from build123d import *

# Parameters (mm, degrees)
SKETCH_2_W          = 80.1
SKETCH_2_H          = 60.1
EXTRUDE_1_DEPTH     = 28
CUT_EXTRUDE_1_DEPTH = 106
SKETCH_6_R          = 1.8
CUT_EXTRUDE_2_DEPTH = 106
CUT_EXTRUDE_3_DEPTH = 92
FILLET_2_R          = 2
FILLET_3_R          = 10
FILLET_4_R          = 2


with BuildPart() as part:
    # 草图2 → 凸台-拉伸1 (new body)
    with BuildSketch(Plane.XY):
        with Locations((40.05, -30.05)):
            Rectangle(SKETCH_2_W, SKETCH_2_H)
    extrude(amount=EXTRUDE_1_DEPTH)

    # 草图3 → 切除-拉伸1 (cut)
    with BuildSketch(Plane.ZY):
        with BuildLine():
            ThreePointArc((14, -22), (6.928932188, -24.928932188), (4, -32))
            Line((4, -32), (14, -32))
            Line((14, -32), (14, -22))
        make_face()
        with BuildLine():
            Line((14, -32), (4, -32))
            ThreePointArc((4, -32), (6.928932188, -39.071067812), (14, -42))
            Line((14, -42), (14, -32))
        make_face()
        with BuildLine():
            Line((14, -22), (14, -32))
            Line((14, -32), (24, -32))
            ThreePointArc((24, -32), (21.071067812, -24.928932188), (14, -22))
        make_face()
        with BuildLine():
            Line((24, -32), (14, -32))
            Line((14, -32), (14, -42))
            ThreePointArc((14, -42), (21.071067812, -39.071067812), (24, -32))
        make_face()
    extrude(amount=-CUT_EXTRUDE_1_DEPTH, mode=Mode.SUBTRACT)

    # 草图6 → 切除-拉伸2 (cut)
    with BuildSketch(Plane.XY.offset(28)):
        with Locations((21.05, -3)):
            Circle(SKETCH_6_R)
        with Locations((59.05, -3)):
            Circle(SKETCH_6_R)
        with Locations((10.05, -54.5)):
            Circle(SKETCH_6_R)
        with Locations((70.05, -54.5)):
            Circle(SKETCH_6_R)
    extrude(amount=-CUT_EXTRUDE_2_DEPTH, mode=Mode.SUBTRACT)

    # 草图9 → 切除-拉伸3 (cut)
    with BuildSketch(Plane(origin=(0, 0, 0), x_dir=(1, 0, 0), z_dir=(0, 1, 0))):
        Polygon((0, 0), (0, -11.5), (25.05, -11.5), (25.05, -16.5), (55.05, -16.5), (55.05, -11.5), (80.1, -11.5), (80.1, 0), align=None)
    extrude(amount=-CUT_EXTRUDE_3_DEPTH, mode=Mode.SUBTRACT)

    # 圆角2
    fillet_2_edges = [part.edges().sort_by_distance(p)[0] for p in [
        (55.05, -50.891229183, 11.5),
        (55.05, -11.158770817, 11.5),
        (55.05, -50.891229183, 16.5),
        (55.05, -11.158770817, 16.5),
        (25.05, -50.891229183, 16.5),
        (25.05, -11.158770817, 16.5),
        (25.05, -50.891229183, 11.5),
        (25.05, -11.158770817, 11.5),
    ]]
    fillet(fillet_2_edges, radius=FILLET_2_R)

    # 圆角3
    fillet_3_edges = [part.edges().sort_by_distance(p)[0] for p in [
        (80.1, -60.1, 19.75),
        (0, -60.1, 19.75),
        (0, 0, 19.75),
        (80.1, 0, 19.75),
    ]]
    fillet(fillet_3_edges, radius=FILLET_3_R)

    # 圆角4
    # the kernel refuses this fillet: 2 mm, written as the material it takes off along each edge
    with BuildSketch(Plane(origin=(0, -50.1, 28), x_dir=(0, 0, -1), z_dir=(0, 1, 0))) as fillet_4_piece_1:
        with BuildLine():
            CenterArc((FILLET_4_R, -FILLET_4_R), FILLET_4_R, 90, 90)
            Line((0, -FILLET_4_R), (0, 0))
            Line((0, 0), (FILLET_4_R, 0))
        make_face()
    extrude(amount=40.1, mode=Mode.SUBTRACT)
    with BuildSketch(Plane(origin=(10, 0, 28), x_dir=(0, -1, 0), z_dir=(1, 0, 0))) as fillet_4_piece_2:
        with BuildLine():
            CenterArc((FILLET_4_R, FILLET_4_R), FILLET_4_R, 180, 90)
            Line((0, FILLET_4_R), (0, 0))
            Line((0, 0), (FILLET_4_R, 0))
        make_face()
    extrude(amount=60.1, mode=Mode.SUBTRACT)
    with BuildSketch(Plane(origin=(80.1, -10, 28), x_dir=(-1, 0, 0), z_dir=(0, -1, 0))) as fillet_4_piece_3:
        with BuildLine():
            CenterArc((FILLET_4_R, FILLET_4_R), FILLET_4_R, 180, 90)
            Line((0, FILLET_4_R), (0, 0))
            Line((0, 0), (FILLET_4_R, 0))
        make_face()
    extrude(amount=40.1, mode=Mode.SUBTRACT)
    with BuildSketch(Plane(origin=(70.1, -60.1, 28), x_dir=(0, 0, -1), z_dir=(-1, 0, 0))) as fillet_4_piece_4:
        with BuildLine():
            CenterArc((FILLET_4_R, -FILLET_4_R), FILLET_4_R, 90, 90)
            Line((0, -FILLET_4_R), (0, 0))
            Line((0, 0), (FILLET_4_R, 0))
        make_face()
    extrude(amount=60.1, mode=Mode.SUBTRACT)
    with BuildSketch(Plane(origin=(70.1, -10, 28), x_dir=(1, 0, 0), z_dir=(0, -1, 0))) as fillet_4_piece_5:
        with BuildLine():
            CenterArc((10 - FILLET_4_R, -FILLET_4_R), FILLET_4_R, 0, 90)
            Line((10, -FILLET_4_R), (10, 0))
            Line((10, 0), (10 - FILLET_4_R, 0))
        make_face()
    revolve(axis=Axis((70.1, -10, 28), (0, 0, 1)), revolution_arc=90, mode=Mode.SUBTRACT)
    with BuildSketch(Plane(origin=(70.1, -50.1, 28), x_dir=(1, 0, 0), z_dir=(0, 1, 0))) as fillet_4_piece_6:
        with BuildLine():
            CenterArc((10 - FILLET_4_R, FILLET_4_R), FILLET_4_R, 270, 90)
            Line((10, FILLET_4_R), (10, 0))
            Line((10, 0), (10 - FILLET_4_R, 0))
        make_face()
    revolve(axis=Axis((70.1, -50.1, 28), (0, 0, -1)), revolution_arc=90, mode=Mode.SUBTRACT)
    with BuildSketch(Plane(origin=(10, -50.1, 28), x_dir=(-1, 0, 0), z_dir=(0, 1, 0))) as fillet_4_piece_7:
        with BuildLine():
            CenterArc((10 - FILLET_4_R, -FILLET_4_R), FILLET_4_R, 0, 90)
            Line((10 - FILLET_4_R, 0), (10, 0))
            Line((10, 0), (10, -FILLET_4_R))
        make_face()
    revolve(axis=Axis((10, -50.1, 28), (0, 0, 1)), revolution_arc=90, mode=Mode.SUBTRACT)
    with BuildSketch(Plane(origin=(10, -10, 28), x_dir=(-1, 0, 0), z_dir=(0, -1, 0))) as fillet_4_piece_8:
        with BuildLine():
            CenterArc((10 - FILLET_4_R, FILLET_4_R), FILLET_4_R, 270, 90)
            Line((10, FILLET_4_R), (10, 0))
            Line((10, 0), (10 - FILLET_4_R, 0))
        make_face()
    revolve(axis=Axis((10, -10, 28), (0, 0, -1)), revolution_arc=90, mode=Mode.SUBTRACT)


solid = part.part
Geometry: final body of the model. Coordinates: model frame, mm. A direction names the side the tool comes from. Give positions to 0.01 mm unless a question says otherwise; leave off trailing zeros. Loops run counter-clockwise (first coordinate to the right, second up) from the corner with the lowest first, then second, coordinate; pieces in that order, holes last. Notation, with made-up numbers: (12, -24.5) -> (23, -24.5) arc R23 cw to (23, -13.5) -> close; hole circle Ø11 at (-14, 30.25). An arc over 180 degrees is marked (long way). Put each result on its own line as item: value.
1. Set-up query: faces 5 (the flat face through (0, -26, 23)), 6 (the cylindrical face through (25.62, -51.02, 15.9)). Return all of +Z, -Z, +X, -X, +Y, -Y with unobstructed straight access to the full face (end or side cutting, diameter ignored); none if empty.
Taken from the geometry:
face 5: +Z, -Z, -X, +Y, -Y
face 6: -Z, +Y, -Y
2. Cut plane B-B (x = 40.5). Return the cut outline in (y, z), plus the area to 3 significant figures.
Taken from the geometry:
outline: (-60.1, 16.5) -> (-41.68, 16.5) arc R10 cw to (-22.32, 16.5) -> (0, 16.5) -> (0, 26) arc R2 ccw to (-2, 28) -> (-58.1, 28) arc R2 ccw to (-60.1, 26) -> close
area: 582 mm2
3. Cut plane C-C (y = -16). Return the cut outline in (x, z).
Taken from the geometry:
outline: (0, 11.5) -> (23.05, 11.5) arc R2 ccw to (25.05, 13.5) -> (25.05, 14.5) arc R2 cw to (27.05, 16.5) -> (53.05, 16.5) arc R2 cw to (55.05, 14.5) -> (55.05, 13.5) arc R2 ccw to (57.05, 11.5) -> (80.1, 11.5) -> (80.1, 26) arc R2 ccw to (78.1, 28) -> (2, 28) arc R2 ccw to (0, 26) -> close
4. Pin query (flat end, axial travel): P1, Ø5.5, axis at x = 35, y = -54.5, coming from the -Z side; P2, Ø1, axis at x = 8.5, z = 16, coming from the +Y side; P3, Ø1.1, axis at y = -53.5, z = 14, coming from the +X side. Return the tip coordinate at first contact, or that it passes through.
Taken from the geometry:
P1: stops at z = 16.5
P2: stops at y = -0.05
P3: stops at x = 79.69
5. Cut plane D-D (z = 15.5). Return the cut outline in (x, y).
Taken from the geometry:
outline: (0, -50.1) arc R10 ccw to (10, -60.1) -> (25.32, -60.1) -> (25.32, -41.89) -> (0, -41.89) -> close; (0, -22.11) -> (25.32, -22.11) -> (25.32, 0) -> (10, 0) arc R10 ccw to (0, -10) -> close; (54.78, -60.1) -> (70.1, -60.1) arc R10 ccw to (80.1, -50.1) -> (80.1, -41.89) -> (54.78, -41.89) -> close; (54.78, -22.11) -> (80.1, -22.11) -> (80.1, -10) arc R10 ccw to (70.1, 0) -> (54.78, 0) -> close; hole circle Ø3.6 at (10.05, -54.5); hole circle Ø3.6 at (21.05, -3); hole circle Ø3.6 at (59.05, -3); hole circle Ø3.6 at (70.05, -54.5)
6. Ray query, line 1 along Y through (x, z) = (59.05, 16.5); line 2 along X through (y, z) = (-3, 23.75); line 3 along Z through (x, y) = (27.5, -11). Return the intervals inside material, ascending. Write a range as [from, to].
Taken from the geometry:
line 1: y = [-60.1, -41.68], [-22.32, -4.8], [-1.2, 0]
line 2: x = [2.86, 19.25], [22.85, 57.25], [60.85, 77.24]
line 3: z = [16.5, 28]
7. Cut plane A-A (z = 19.5). Return the cut outline in (x, y), plus the area to 3 significant figures.
Taken from the geometry:
outline: (0, -50.1) arc R10 ccw to (10, -60.1) -> (70.1, -60.1) arc R10 ccw to (80.1, -50.1) -> (80.1, -40.35) -> (0, -40.35) -> close; (0, -23.65) -> (80.1, -23.65) -> (80.1, -10) arc R10 ccw to (70.1, 0) -> (10, 0) arc R10 ccw to (0, -10) -> close; hole circle Ø3.6 at (10.05, -54.5); hole circle Ø3.6 at (21.05, -3); hole circle Ø3.6 at (59.05, -3); hole circle Ø3.6 at (70.05, -54.5)
area: 3,350 mm2
8. Pull-direction query (X, two-part tool) for faces 1 (the flat face through (68, -11, 11.5)), 2 (the flat face through (40, -11, 16.5)), 3 (the cylindrical face through (9.816, -52.715, 19.866)), 4 (the cylindrical face through (77.09, -57.25, 18.85)); classes: released by +X, released by -X, zero draft, split by the parting line, or undercut.
Taken from the geometry:
face 1: zero draft
face 2: undercut
face 3: undercut
face 4: released by +X
